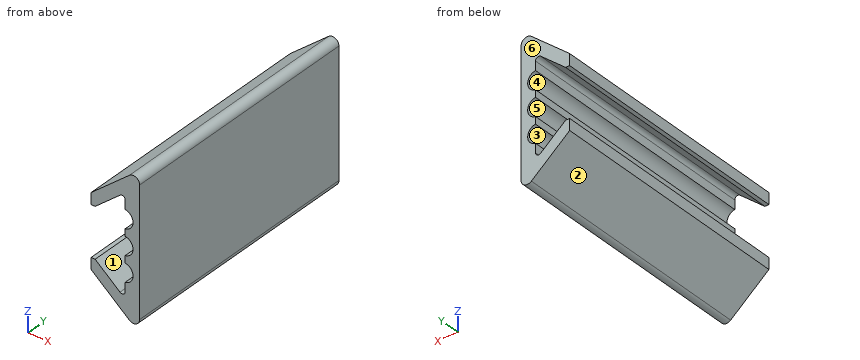
from build123d import *

# Parameters (mm, degrees)
BOSS_EXTRUDE1_DEPTH = 80


with BuildPart() as part:
    # Sketch1 → Boss-Extrude1 (new body)
    with BuildSketch(Plane(origin=(0, 0, 0), x_dir=(1, 0, 0), z_dir=(0, 1, 0))):
        with BuildLine():
            Line((18.551800259, 11.5), (18.551800259, 7.9))
            Line((18.551800259, 7.9), (19.855180026, 7.9))
            Line((19.855180026, 7.9), (27.7598156, 14.487196312))
            ThreePointArc((27.7598156, 14.487196312), (28.824155396, 14.624564454), (29.4, 13.718975032))
            Line((29.4, 13.718975032), (29.4, 10.872281323))
            ThreePointArc((29.4, 10.872281323), (31.9, 8), (29.4, 5.127718677))
            Line((29.4, 5.127718677), (29.4, 2.872281323))
            ThreePointArc((29.4, 2.872281323), (31.9, 0), (29.4, -2.872281323))
            Line((29.4, -2.872281323), (29.4, -5.127718677))
            ThreePointArc((29.4, -5.127718677), (31.9, -8), (29.4, -10.872281323))
            Line((29.4, -10.872281323), (29.4, -13.718975032))
            ThreePointArc((29.4, -13.718975032), (28.824155396, -14.624564454), (27.7598156, -14.487196312))
            Line((27.7598156, -14.487196312), (19.845818206, -7.892198484))
            Line((19.845818206, -7.892198484), (18.551800259, -7.892198484))
            Line((18.551800259, -7.892198484), (18.551800259, -11.5))
            Line((18.551800259, -11.5), (30.719631201, -21.639859118))
            ThreePointArc((30.719631201, -21.639859118), (32.848310792, -21.914595401), (34, -20.103416559))
            Line((34, -20.103416559), (34, 20.103416559))
            ThreePointArc((34, 20.103416559), (32.848310792, 21.914595401), (30.719631201, 21.639859118))
            Line((30.719631201, 21.639859118), (18.551800259, 11.5))
        make_face()
    extrude(amount=BOSS_EXTRUDE1_DEPTH)


solid = part.part
CAD build for the part. Positions are in the model's coordinates, mm. Face numbers are marked on the shaded views. A direction names the side the tool comes from. Give positions to 0.01 mm unless a question says otherwise; leave off trailing zeros. Order: outer loops, then holes, each group sorted by start corner. A loop starts at its lowest first (then second) coordinate and runs counter-clockwise, first axis right, second up. Notation, with made-up numbers: (84, -6) -> (100, -6) arc R33 ccw to (100, 30) -> close; hole circle Ø7 at (-12.5, 71.25). An arc over 180 degrees is marked (long way). Return JSON: item names as keys, results as strings.
Q1. Saw through at D-D (z = 6.5). Write the cut outline in (x, y).
Working result:
{"outline": "(31.48, 0) -> (34, 0) -> (34, 80) -> (31.48, 80) -> close"}
Q2. Saw through at A-A (x = 22.25). Write the cut outline in (y, z), then the cut area to 3 significant figures.
Working result:
{"outline": "(0, -14.58) -> (80, -14.58) -> (80, -9.9) -> (0, -9.9) -> close; (0, 9.9) -> (80, 9.9) -> (80, 14.58) -> (0, 14.58) -> close", "area": "750 mm²"}
Q3. Flat gauge pins, fed straight in: pin 1 (2.5 mm diameter, centred on y = 49, z = -12.5, fed in from -X); pin 2 (1.8 mm diameter, centred on y = 28.5, z = -4, fed in from -X); pin 3 (0.7 mm diameter, centred on x = 19, y = 49, fed in from +Z); pin 4 (0.6 mm diameter, centred on x = 19, y = 46, fed in from -Z). Where does each tip first touch, or does it go through?
Working result:
{"pin 1": "x = 18.55", "pin 2": "x = 29.4", "pin 3": "z = 12.17", "pin 4": "z = -12.12"}
Q4. Saw through at B-B (y = 22.5). Write the cut outline in (x, z), then the cut area to 3 significant figures.
Working result:
{"outline": "(18.55, -11.5) -> (30.72, -21.64) arc R2 ccw to (34, -20.1) -> (34, 20.1) arc R2 ccw to (30.72, 21.64) -> (18.55, 11.5) -> (18.55, 7.89) -> (19.85, 7.89) -> (27.76, 14.49) arc R1 cw to (29.4, 13.72) -> (29.4, 10.87) arc R2.9 cw to (29.4, 5.13) -> (29.4, 2.87) arc R2.9 cw to (29.4, -2.87) -> (29.4, -5.13) arc R2.9 cw to (29.4, -10.87) -> (29.4, -13.72) arc R1 cw to (27.76, -14.49) -> (19.86, -7.9) -> (18.55, -7.9) -> close", "area": "268 mm²"}
Q5. Which spindle directions (+Z, -Z, +X, -X, +Y, -Y) get a long thin tool onto all of the face, cutting with end or side? Do the marked faces 1 and 2. Say none if no direction does.
Working result:
{"face 1": "+Y, -Y", "face 2": "-Z, -X, +Y, -Y"}
Q6. Mould opens along X. For the marked faces 3, 4, 5 and 6 say: pulls with the +X half, pulls with the -X half, needs draft (parallel to the pull), parting line crosses it, or undercut.
Working result:
{"face 3": "undercut", "face 4": "undercut", "face 5": "pulls with the -X half", "face 6": "needs draft"}
Q7. Drill centre lines: line 1 (X direction, y = 25, z = 0); line 2 (Z direction, x = 30.5, y = 25); line 3 (Z direction, x = 26, y = 29.5). Where is each one in solid material? Low to high.
Working result:
{"line 1": "31.9 to 34", "line 2": "-21.46 to -10.48, -5.52 to -2.48, 2.48 to 5.52, 10.48 to 21.46", "line 3": "-17.71 to -13.02, 13.02 to 17.71"}
Q8. Saw through at C-C (z = 18). Write the cut outline in (x, y).
Working result:
{"outline": "(26.35, 0) -> (34, 0) -> (34, 80) -> (26.35, 80) -> close"}
